```python
from build123d import *

# Parameters (mm, degrees)
EXTRUDE_1_DEPTH = 3


with BuildPart() as part:
    # 草图1 → 凸台-拉伸1 (new body)
    with BuildSketch(Plane.XY):
        with BuildLine():
            Line((28.2, -17.2), (28.2, 17.2))
            ThreePointArc((28.2, 17.2), (27.614213562, 18.614213562), (26.2, 19.2))
            Line((26.2, 19.2), (23.2, 19.2))
            ThreePointArc((23.2, 19.2), (20.371572875, 20.371572875), (19.2, 23.2))
            Line((19.2, 23.2), (19.2, 26.2))
            ThreePointArc((19.2, 26.2), (18.614213562, 27.614213562), (17.2, 28.2))
            Line((17.2, 28.2), (-17.2, 28.2))
            ThreePointArc((-17.2, 28.2), (-18.614213562, 27.614213562), (-19.2, 26.2))
            Line((-19.2, 26.2), (-19.2, 23.2))
            ThreePointArc((-19.2, 23.2), (-20.371572875, 20.371572875), (-23.2, 19.2))
            Line((-23.2, 19.2), (-26.2, 19.2))
            ThreePointArc((-26.2, 19.2), (-27.614213562, 18.614213562), (-28.2, 17.2))
            Line((-28.2, 17.2), (-28.2, -17.2))
            ThreePointArc((-28.2, -17.2), (-27.614213562, -18.614213562), (-26.2, -19.2))
            Line((-26.2, -19.2), (-23.2, -19.2))
            ThreePointArc((-23.2, -19.2), (-20.371572875, -20.371572875), (-19.2, -23.2))
            Line((-19.2, -23.2), (-19.2, -26.2))
            ThreePointArc((-19.2, -26.2), (-18.614213562, -27.614213562), (-17.2, -28.2))
            Line((-17.2, -28.2), (17.2, -28.2))
            ThreePointArc((17.2, -28.2), (18.614213562, -27.614213562), (19.2, -26.2))
            Line((19.2, -26.2), (19.2, -23.2))
            ThreePointArc((19.2, -23.2), (20.371572875, -20.371572875), (23.2, -19.2))
            Line((23.2, -19.2), (26.2, -19.2))
            ThreePointArc((26.2, -19.2), (27.614213562, -18.614213562), (28.2, -17.2))
        make_face()
    extrude(amount=EXTRUDE_1_DEPTH)


solid = part.part
```
Check sheet for the modelled part. Datum: model origin and axes. Units: mm. A direction names the side the tool comes from. Give positions to 0.01 mm unless a question says otherwise; leave off trailing zeros. Order: outer loops, then holes, each group sorted by start corner. A loop starts at its lowest first (then second) coordinate and runs counter-clockwise, first axis right, second up. Notation, with made-up numbers: (88, -11.75) -> (104, -11.75) arc R8 ccw to (104, -0.75) -> close; hole circle Ø8 at (49, 66). An arc over 180 degrees is marked (long way). Use CSV: the item, a comma, the result in double quotes. Start each with the question number.
1) Set-up check for faces 1 (the face through (25, -19.2, 1)), 2 (the face through (25, 19.2, 1)), 3 (the face through (-19.2, -25, 1)), 4 (the face through (-25, 19.2, 1)): record each of +Z, -Z, +X, -X, +Y, -Y from which the full face is reachable in a straight line by a thin tool's end or side.
2) Material ranges on line 1 (X direction, y = 23.5, z = 1.5); line 2 (Y direction, x = 22, z = 0.3), recorded low to high. Write a range as from..to.
3) Sectioned sample at A-A, the plane z = 0.45. Record the boundary of the cut face in (x, y), plus the area to 3 significant figures.
4) Sectioned sample at B-B, the plane x = -20. Record the boundary of the cut face in (y, z), plus the area to 3 significant figures.
5) Sectioned sample at C-C, the plane x = 20.5. Record the boundary of the cut face in (y, z), plus the area to 3 significant figures.
6) Go/stop test with flat-tipped pins: P1, Ø1.5, axis at x = 24, z = 2, coming from the -Y side; P2, Ø1.5, axis at y = -24.5, z = 2, coming from the +X side; P3, Ø1.5, axis at y = 25.5, z = 2, coming from the -X side. Record where each tip stops, or that it passes through.
Recorded:
1,face 1,"+Z, -Z, +X, -Y"
1,face 2,"+Z, -Z, +X, +Y"
1,face 3,"+Z, -Z, -X, -Y"
1,face 4,"+Z, -Z, -X, +Y"
2,line 1,"-19.2..19.2"
2,line 2,"-19.38..19.38"
3,outline,"(-28.2, -17.2) arc R2 ccw to (-26.2, -19.2) -> (-23.2, -19.2) arc R4 cw to (-19.2, -23.2) -> (-19.2, -26.2) arc R2 ccw to (-17.2, -28.2) -> (17.2, -28.2) arc R2 ccw to (19.2, -26.2) -> (19.2, -23.2) arc R4 cw to (23.2, -19.2) -> (26.2, -19.2) arc R2 ccw to (28.2, -17.2) -> (28.2, 17.2) arc R2 ccw to (26.2, 19.2) -> (23.2, 19.2) arc R4 cw to (19.2, 23.2) -> (19.2, 26.2) arc R2 ccw to (17.2, 28.2) -> (-17.2, 28.2) arc R2 ccw to (-19.2, 26.2) -> (-19.2, 23.2) arc R4 cw to (-23.2, 19.2) -> (-26.2, 19.2) arc R2 ccw to (-28.2, 17.2) -> close"
3,area,"2,860 mm2"
4,outline,"(-20.8, 0) -> (20.8, 0) -> (20.8, 3) -> (-20.8, 3) -> close"
4,area,"125 mm2"
5,outline,"(-20.25, 0) -> (20.25, 0) -> (20.25, 3) -> (-20.25, 3) -> close"
5,area,"121 mm2"
6,P1,"y = -19.2"
6,P2,"x = 19.2"
6,P3,"x = -19.2"
